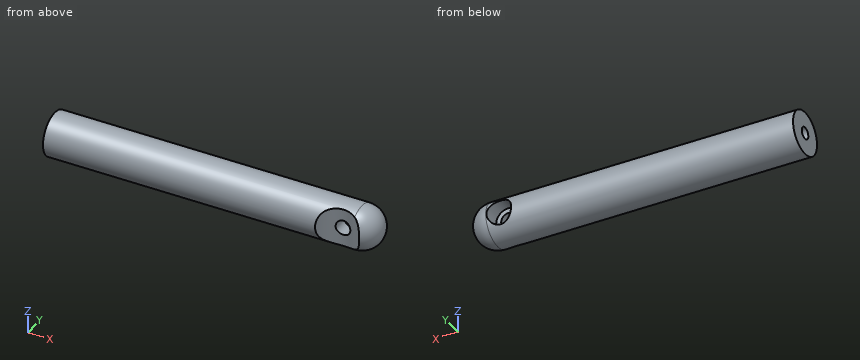
```python
from build123d import *

# Parameters (mm, degrees)
F3_R           = 16
F4_DEPTH       = 15
F6_D           = 6.8
F6_DEPTH       = 23.75
F6_TIP         = 2.0429261047
F9_D           = 8.5
F9_START       = 2.2294414
F9_CBORE_D     = 14.25
F9_CBORE_DEPTH = 8


with BuildPart() as f2:
    # F0 (on Top) → F2 (revolve)
    with BuildSketch(Plane.XY):
        with BuildLine():
            Line((0, 12.5), (0, 0))
            Line((0, 0), (190, 0))
            ThreePointArc((190, 0), (186.3388347648, 8.8388347648), (177.5, 12.5))
            Line((177.5, 12.5), (0, 12.5))
        make_face()
    revolve(axis=Axis((6.2984433025, 0, 0), (-1, 0, 0)))

    # F3 (on Top) → F4 (cut, symmetric)
    with BuildSketch(Plane.XY):
        with Locations((170, -22)):
            Circle(F3_R)
    extrude(amount=F4_DEPTH, both=True, mode=Mode.SUBTRACT)

    # F6
    with Locations(Plane(origin=(0, 0, 0), x_dir=(0, 1, 0), z_dir=(-1, 0, 0))):
        with Locations((0, 0)):
            Hole(F6_D / 2, depth=F6_DEPTH)
            with Locations((0, 0, -(F6_DEPTH + F6_TIP / 2))):  # 118° drill point
                Cone(0, F6_D / 2, F6_TIP, mode=Mode.SUBTRACT)

    # F9 (through all)
    # its depths count from where the whole tool has entered the part; down to there all is cleared
    with Locations(Plane(origin=(0, 12.5, 0), x_dir=(1, 0, 0), z_dir=(0, 1, 0)).offset(-F9_START)):
        with Locations((170, 0)):
            CounterBoreHole(F9_D / 2, F9_CBORE_D / 2, F9_CBORE_DEPTH)


solid = f2.part
```
Build history of the part. All positions in model axes, mm. Give positions to 0.01 mm unless a question says otherwise; leave off trailing zeros. Order: outer loops, then holes, each group sorted by start corner. A loop starts at its lowest first (then second) coordinate and runs counter-clockwise, first axis right, second up. Notation, with made-up numbers: M -22.5,11 L 11.5,11 A27 cw 11.5,45 Z; hole C -14.75,-38 d11. An arc over 180 degrees is marked long. Return JSON: item names as keys, results as strings.
Q1. Wall check: probe 1 along Z at (x, y) = (16, 0); probe 2 along X at (y, z) = (-8.25, -1); probe 3 along X at (y, z) = (9.75, -4). Give the ranges that are in metal, low to high. Write a range as from..to.
Answer list:
{"probe 1": "z = -12.5..-3.4, 3.4..12.5", "probe 2": "x = 0..161.82, 178.18..186.84", "probe 3": "x = 0..164.1, 175.9..184.22"}
Q2. Band-saw the part on A-A (x = 170). Give the cut face in (y, z) (3 decimals).
Answer list:
{"outline": "M -6,-10.966 A12.5 ccw 10.271,-7.125 L 2.271,-7.125 L 2.271,-4.25 L -6,-4.25 Z; M -6,4.25 L 2.271,4.25 L 2.271,7.125 L 10.271,7.125 A12.5 ccw -6,10.966 Z"}
Q3. Band-saw the part on C-C (x = 97.5). Give the cut face in (y, z).
Answer list:
{"outline": "C 0,0 d25"}
Q4. Band-saw the part on B-B (y = 10.25). Give the cut face in (x, z) (3 decimals).
Answer list:
{"outline": "M 0,-7.155 L 177.5,-7.155 A7.155 ccw 177.5,7.155 L 0,7.155 Z; hole C 170,0 d14.25"}
Q5. Flat gauge pins, fed straight in: pin 1 (2 mm diameter, centred on x = 41, z = -9, fed in from +Y); pin 2 (4 mm diameter, centred on x = 171, y = 3, fed in from -Z); pin 3 (8 mm diameter, centred on x = 115, y = -4.5, fed in from +Z). Where does each tip first touch, or does it go through?
Answer list:
{"pin 1": "stops at y = 9.6", "pin 2": "stops at z = -12.46", "pin 3": "stops at z = 12.49"}
